Part model, mm, in its own coordinate system. A direction names the side the tool comes from. Coordinates: 2 decimals unless noted, no trailing zeros. Write each loop counter-clockwise with the first axis right and the second up, starting at its lowest first coordinate (ties: lowest second). Pieces come first, ordered by that corner, then holes. Notation, with made-up numbers: M -21.75,21 L 2.25,21 A35 cw 2.25,58 Z; hole C -28.5,47 d8. An arc over 180 degrees is marked long. Use a Markdown table: item, result. Add a question column.
Q1. Slice it at A-A on y = -5.25. Write the cut outline in (x, z).
Q2. Mould opens along X. For faces 4 (the flat face through (1.8, -10, 6.5)), 5 (the flat face through (1.901, -4.93, 5.965)), 6 (the flat face through (0, -8, 0)) say: released by +X, released by -X, zero draft, split by the parting line, or undercut.
Q3. Pin check, flat tips, straight feed: pin 1 Ø8 at (y, z) = (-0.5, 6.5) entering from +X; pin 2 Ø2.5 at (x, y) = (-7.5, -4.5) entering from +Z; pin 3 Ø0.9 at (x, z) = (0.5, 0) entering from +Y; pin 4 Ø1 at (y, z) = (-1, 9.5) entering from +X. Stop position of each tip, or through.
Q4. Wall check: L1, parallel to Z at x = 0, y = 0.05; L2, parallel to Y at x = 8.75, z = 5; L3, parallel to Y at x = 7.25, z = 0.25. Give the ranges that are in metal, low to high. Write a range as from..to.
Q5. Slice it at B-B on z = 7.75. Write the cut outline in (x, y), then the cut area to 3 significant figures.
Q6. Slice it at D-D on z = 9.5. Write the cut outline in (x, y).
Q7. Tool access for faces 1 (the flat face through (-1.849, -4.93, 6.035)), 2 (the flat face through (-8.3, -10.5, 5.5)), 3 (the flat face through (8.4, -10.5, 5.5)): list every direction of +Z, -Z, +X, -X, +Y, -Y with a clear straight run to the whole face (end or side of a thin tool).
Q8. Slice it at C-C on x = 9. Write the cut outline in (y, z), then the cut area to 3 significant figures.
from build123d import *

# Parameters (mm, degrees)
F0_R     = 1.5
F1_DEPTH = 10
F4_DEPTH = 4
F2_R     = 1.5
F5_DEPTH = 2
F6_R     = 1.5
F7_DEPTH = 0.02
F9_DEPTH = 1


with BuildPart() as f1:
    # F0 (on Front) → F1 (new body)
    with BuildSketch(Plane.XZ):
        with BuildLine():
            Line((-3.75, 3.5), (-12.678722, 3.5))
            ThreePointArc((-12.678722, 3.5), (-12.861248, 2.754688), (-13, 2))
            Line((-13, 2), (-1.581139, -1.806287))
            ThreePointArc((-1.581139, -1.806287), (0, -2.062871), (1.581139, -1.806287))
            Line((1.581139, -1.806287), (13, 2))
            ThreePointArc((13, 2), (12.861248, 2.754688), (12.678722, 3.5))
            Line((12.678722, 3.5), (3.75, 3.5))
            Line((3.75, 3.5), (0, 8.5))
            Line((0, 8.5), (-3.75, 3.5))
        make_face()
        Circle(F0_R, mode=Mode.SUBTRACT)
    extrude(amount=F1_DEPTH)

    # F3 (on face) → F4 (join)
    with BuildSketch(Plane(origin=(0, 0, 0), x_dir=(-1, 0, 0), z_dir=(0, 1, 0))):
        with BuildLine():
            Line((0, 3.5), (0, 5.75))
            ThreePointArc((0, 5.75), (-1.125, 4.625), (0, 3.5))
        make_face()
        with BuildLine():
            ThreePointArc((0, 3.5), (0.795495, 3.829505), (1.125, 4.625))
            ThreePointArc((1.125, 4.625), (0.795495, 5.420495), (0, 5.75))
            Line((0, 5.75), (0, 3.5))
        make_face()
    extrude(amount=F4_DEPTH)

    # F2 (on face) → F5 (join)
    with BuildSketch(Plane.XZ.offset(10)):
        Circle(F2_R)
    extrude(amount=-F5_DEPTH)

    # F6 (on face) → F7 (join)
    with BuildSketch(Plane(origin=(0, 0, 0), x_dir=(-1, 0, 0), z_dir=(0, 1, 0))):
        with BuildLine():
            ThreePointArc((0, -2), (1.414214, -1.414214), (2, 0))
            ThreePointArc((2, 0), (-1.414214, 1.414214), (0, -2))
        make_face()
        Circle(F6_R, mode=Mode.SUBTRACT)
    extrude(amount=F7_DEPTH)

    # F8 (on face) → F9 (join)
    with BuildSketch(Plane.XZ.offset(10)):
        with BuildLine():
            Line((0, 11.833333), (-4.75, 5.5))
            Line((-4.75, 5.5), (-11.947803, 5.5))
            ThreePointArc((-11.947803, 5.5), (-12.353803, 4.514816), (-12.678722, 3.5))
            Line((-12.678722, 3.5), (-3.75, 3.5))
            Line((-3.75, 3.5), (0, 8.5))
            Line((0, 8.5), (3.75, 3.5))
            Line((3.75, 3.5), (12.678722, 3.5))
            ThreePointArc((12.678722, 3.5), (12.353803, 4.514816), (11.947803, 5.5))
            Line((11.947803, 5.5), (4.75, 5.5))
            Line((4.75, 5.5), (0, 11.833333))
        make_face()
        with BuildLine():
            Line((-3.75, 3.5), (-12.678722, 3.5))
            ThreePointArc((-12.678722, 3.5), (-12.861248, 2.754688), (-13, 2))
            Line((-13, 2), (-1.581139, -1.806287))
            ThreePointArc((-1.581139, -1.806287), (0, -2.062871), (1.581139, -1.806287))
            Line((1.581139, -1.806287), (13, 2))
            ThreePointArc((13, 2), (12.861248, 2.754688), (12.678722, 3.5))
            Line((12.678722, 3.5), (3.75, 3.5))
            Line((3.75, 3.5), (0, 8.5))
            Line((0, 8.5), (-3.75, 3.5))
        make_face()
    extrude(amount=F9_DEPTH)


solid = f1.part
Recorded:
| question | item | result |
|---|---|---|
| 1 | outline | M -13,2 L -1.58,-1.81 A5 ccw 1.58,-1.81 L 13,2 A13.15 ccw 12.68,3.5 L 3.75,3.5 L 0,8.5 L -3.75,3.5 L -12.68,3.5 A13.15 ccw Z; hole C 0,0 d3 |
| 2 | face 4 | zero draft |
| 2 | face 5 | released by +X |
| 2 | face 6 | undercut |
| 3 | pin 1 | x = 12.91 |
| 3 | pin 2 | z = 3.5 |
| 3 | pin 3 | y = -8 |
| 3 | pin 4 | through |
| 4 | L1 | 3.5..5.75 |
| 4 | L2 | -11..-10 |
| 4 | L3 | -11..0 |
| 5 | outline | M -3.06,-11 L 3.06,-11 L 3.06,-10 L 0.56,-10 L 0.56,0 L -0.56,0 L -0.56,-10 L -3.06,-10 Z |
| 5 | area | 17.4 mm² |
| 6 | outline | M -1.75,-11 L 1.75,-11 L 1.75,-10 L -1.75,-10 Z |
| 7 | face 1 | +Z, -X, +Y |
| 7 | face 2 | +Z, -X, +Y, -Y |
| 7 | face 3 | +Z, +X, +Y, -Y |
| 8 | outline | M -11,0.67 L 0,0.67 L 0,3.5 L -10,3.5 L -10,5.5 L -11,5.5 Z |
| 8 | area | 33.2 mm² |
